Part model, mm, in its own coordinate system. A direction names the side the tool comes from. Round coordinates to 2 decimals unless told otherwise and drop trailing zeros. Loops run counter-clockwise (first coordinate to the right, second up) from the corner with the lowest first, then second, coordinate; pieces in that order, holes last.
1) Mould opens along Y. For faces 1 (the cylindrical face through (-3.853, 0.018, -12.235)), 2 (the flat face through (8.5, 29.21, 5)), 3 (the flat face through (0, 0, 0)) say: +Y half, -Y half, draft (parallel to the pull), parting line (faces both ways), or undercut.
2) Probe line 1 (X direction, y = 23.5, z = 0) (3 decimals); line 2 (X direction, y = -0.7, z = 0); line 3 (Y direction, x = 4, z = 1.5) (3 decimals). List the from-to ranges inside material, lowest first.
3) Band-saw the part on D-D, the plane y = 3. Write the cut outline in (x, z).
4) Drop flat-ended pins along their axis: P1, Ø12, axis at x = 9, y = 21, coming from the -Z side; P2, Ø2, axis at y = 12.5, z = 10, coming from the +X side; P3, Ø1, axis at y = 19, z = 5.5, coming from the +X side. Give the stop position or say it passes through.
5) Band-saw the part on C-C, the plane y = 27.5. Write the cut outline in (x, z) (3 decimals), then the cut area to 3 significant figures.
6) 3-axis set-ups, long thin cutter, end or side, ignore diameter. For faces 4 (the flat face through (-8.5, 29.21, -4.7)), 5 (the cylindrical face through (-2.33, 37.54, -7.39)), 6 (the flat face through (8.6, 29.21, -5)), 7 (the flat face through (0, 31, 9.459)), 8 (the flat face through (8.16, 30.82, 4.78)): which of +Z, -Z, +X, -X, +Y, -Y reach the whole face in a straight line?
7) Band-saw the part on B-B, the plane z = 0. Write the cut outline in (x, y) (3 decimals), then the cut area to 3 significant figures.
8) Band-saw the part on A-A, the plane x = 0. Write the cut outline in (y, z) (3 decimals).
from build123d import *

# Parameters (mm, degrees)
SKETCH2_R               = 12.827
CUT_EXTRUDE1_DEPTH      = 3.175
CUT_EXTRUDE2_DEPTH      = 48.421704767
CUT_EXTRUDE2_DEPTH_BACK = 33.02
SKETCH3_R               = 1.905


with BuildPart() as part:
    # Sketch1 → Revolve1 (revolve)
    with BuildSketch(Plane.XY, mode=Mode.PRIVATE) as revolve1_sk:
        Polygon((0, 0), (11.557, 0), (11.557, -1.27), (12.827, -1.27), (12.827, 1.27), (10.922, 1.27), (10.922, 24.13), (10.287, 24.765), (10.287, 32.385), (7.747, 32.385), (7.747, 42.545), (0, 42.545), (0, 32.385), align=None)
    revolve(revolve1_sk.sketch.rotate(Axis((0, 0, 0), (0, 1, 0)), 90), axis=Axis((0, 0, 0), (0, 1, 0)))

    # Sketch2 → Cut-Extrude1 (cut)
    with BuildSketch(Plane(origin=(0, 32.385, 0), x_dir=(1, 0, 0), z_dir=(0, 1, 0))):
        with Locations(Location((0, 0, 0), (0, 0, 90))):
            Circle(SKETCH2_R)
        Polygon((-10.922, 0), (-5.461, -9.45872946), (5.461, -9.45872946), (10.922, 0), (5.461, 9.45872946), (-5.461, 9.45872946), align=None, mode=Mode.SUBTRACT)
    extrude(amount=-CUT_EXTRUDE1_DEPTH, mode=Mode.SUBTRACT)

    # Sketch3 → Cut-Extrude2 (cut, two sides: drawn at the far end of the back side and taken through both)
    with BuildSketch(Plane(origin=(0, 42.545, 0), x_dir=(1, 0, 0), z_dir=(0, 1, 0)).offset(-CUT_EXTRUDE2_DEPTH_BACK)):
        with Locations(Location((0, 0, 0), (0, 0, 90))):
            Circle(SKETCH3_R)
    extrude(amount=CUT_EXTRUDE2_DEPTH + CUT_EXTRUDE2_DEPTH_BACK, mode=Mode.SUBTRACT)


solid = part.part
Reported:
1. face 1: draft
1. face 2: +Y half
1. face 3: -Y half
2. line 1: x = -10.922 to -1.905, 1.905 to 10.922
2. line 2: x = -12.83 to -11.56, 11.56 to 12.83
2. line 3: y = 0 to 42.545
3. outline: circle Ø21.84 at (0, 0)
4. P1: stops at z = -10.5
4. P2: stops at x = 6.19
4. P3: stops at x = 9.71
5. outline: circle Ø20.574 at (0, 0); hole circle Ø3.81 at (0, 0)
5. area: 321 mm2
6. face 4: -Z, -X, +Y
6. face 5: +Y
6. face 6: -Z, +X, +Y
6. face 7: +Z, +X, -X, +Y
6. face 8: +Z, +X, +Y
7. outline: (-12.827, -1.27) - (-11.557, -1.27) - (-11.557, 0) - (11.557, 0) - (11.557, -1.27) - (12.827, -1.27) - (12.827, 1.27) - (10.922, 1.27) - (10.922, 24.13) - (10.287, 24.765) - (10.287, 32.385) - (7.747, 32.385) - (7.747, 42.545) - (1.905, 42.545) - (1.905, 9.525) - (-1.905, 9.525) - (-1.905, 42.545) - (-7.747, 42.545) - (-7.747, 32.385) - (-10.287, 32.385) - (-10.287, 24.765) - (-10.922, 24.13) - (-10.922, 1.27) - (-12.827, 1.27) - close
7. area: 737 mm2
8. outline: (-1.27, -12.827) - (1.27, -12.827) - (1.27, -10.922) - (24.13, -10.922) - (24.765, -10.287) - (29.21, -10.287) - (29.21, -9.459) - (32.385, -9.459) - (32.385, -7.747) - (42.545, -7.747) - (42.545, -1.905) - (9.525, -1.905) - (9.525, 1.905) - (42.545, 1.905) - (42.545, 7.747) - (32.385, 7.747) - (32.385, 9.459) - (29.21, 9.459) - (29.21, 10.287) - (24.765, 10.287) - (24.13, 10.922) - (1.27, 10.922) - (1.27, 12.827) - (-1.27, 12.827) - (-1.27, 11.557) - (0, 11.557) - (0, -11.557) - (-1.27, -11.557) - close
